```python
from build123d import *

# Parameters (mm, degrees)
EXTRUDE_1_DEPTH = 7.5
SKETCH_2_R      = 6
EXTRUDE_2_DEPTH = 45
CHAMFER_1_SIZE  = 0.828


with BuildPart() as part:
    # Эскиз1 → Бобышка-Вытянуть1 (new body)
    with BuildSketch(Plane.XY):
        Polygon((0, 10.392304845), (-9, 5.196152423), (-9, -5.196152423), (0, -10.392304845), (9, -5.196152423), (9, 5.196152423), align=None)
    extrude(amount=EXTRUDE_1_DEPTH)

    # Эскиз2 → Бобышка-Вытянуть2 (add)
    with BuildSketch(Plane.XY.offset(7.5)):
        Circle(SKETCH_2_R)
    extrude(amount=EXTRUDE_2_DEPTH)

    # Фаска1
    chamfer_1_edges = [part.edges().sort_by_distance(p)[0] for p in [
        (-6, 0, 52.5),
    ]]
    chamfer(chamfer_1_edges, length=CHAMFER_1_SIZE)


solid = part.part
```
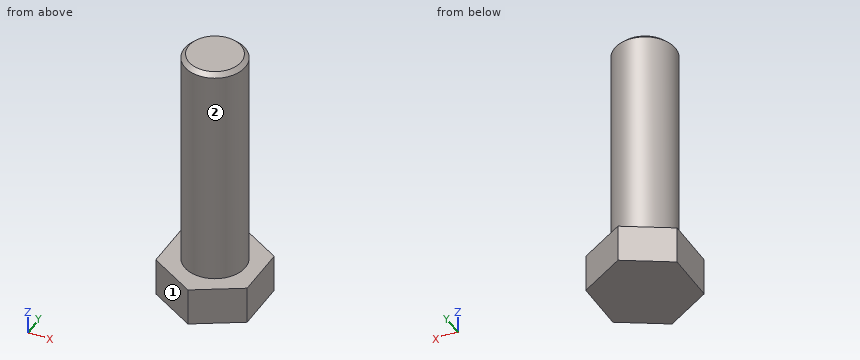
Work out the finished part from the listing and answer in its coordinate system (mm). Face numbers are marked on the shaded views. A direction names the side the tool comes from. Coordinates: 2 decimals unless noted, no trailing zeros. Write each loop counter-clockwise with the first axis right and the second up, starting at its lowest first coordinate (ties: lowest second). Pieces come first, ordered by that corner, then holes. Notation, with made-up numbers: (-8.75, 82) - (19.25, 82) arc R14 ccw to (19.25, 103) - close; hole circle Ø6 at (60.5, 36.5). An arc over 180 degrees is marked (long way). Answer as a JSON object with one key per item and string values.
Q1. Find section D-D (y = -8.25). Write down the section's boundary in (x, z), plus the area to 3 significant figures.
Results list:
{"outline": "(-3.71, 0) - (3.71, 0) - (3.71, 7.5) - (-3.71, 7.5) - close", "area": "55.7 mm^2"}
Q2. Find section B-B (z = 39.5). Write down the section's boundary in (x, y).
Results list:
{"outline": "circle Ø12 at (0, 0)"}
Q3. Given pin 1 Ø5 at (x, y) = (6.5, 6) entering from +Z; pin 2 Ø10 at (x, z) = (0, 13) entering from -Y; pin 3 Ø2 at (y, z) = (6, 12) entering from +X, each flat-ended and moving along its own axis, determine where each tip first touches the part or whether it passes through.
Results list:
{"pin 1": "stops at z = 7.5", "pin 2": "stops at y = -6", "pin 3": "stops at x = 3.32"}
Q4. Which of the six approach directions +Z, -Z, +X, -X, +Y, -Y give full straight-line access (tool end or side, diameter ignored) to the marked faces 1 and 2?
Results list:
{"face 1": "+Z, -Z, -X, -Y", "face 2": "+Z"}
Q5. Find section C-C (x = -7.5). Write down the section's boundary in (y, z), plus the area to 3 significant figures.
Results list:
{"outline": "(-6.06, 0) - (6.06, 0) - (6.06, 7.5) - (-6.06, 7.5) - close", "area": "90.9 mm^2"}
Q6. Consider L1, parallel to X at y = 3, z = 12.5; L2, parallel to Z at x = 6.5, y = 4.25; L3, parallel to Y at x = -3.75, z = 8. Determine where each line is inside the solid, lowest interval first. Write a range as from..to.
Results list:
{"L1": "x = -5.2..5.2", "L2": "z = 0..7.5", "L3": "y = -4.68..4.68"}
Q7. Find section A-A (y = 0). Write down the section's boundary in (x, z), plus the area to 3 significant figures.
Results list:
{"outline": "(-9, 0) - (9, 0) - (9, 7.5) - (6, 7.5) - (6, 51.67) - (5.17, 52.5) - (-5.17, 52.5) - (-6, 51.67) - (-6, 7.5) - (-9, 7.5) - close", "area": "674 mm^2"}
